Could you check a few things on this model? Use its own coordinates, in mm. Face numbers are marked on the shaded views. A direction names the side the tool comes from. Round coordinates to 2 decimals unless told otherwise and drop trailing zeros. Write each loop counter-clockwise with the first axis right and the second up, starting at its lowest first coordinate (ties: lowest second). Pieces come first, ordered by that corner, then holes. Notation, with made-up numbers: M -18,-2.75 L 10,-2.75 A29 cw 10,18.25 Z; hole C 24.5,-3.75 d10. An arc over 180 degrees is marked long. One line per question, with ' | ' between items. Start each with the question number.
```python
from build123d import *

# Parameters (mm, degrees)
F2_R    = 0.5
F3_R    = 0.9
F4_SIZE = 0.5


with BuildPart() as f1:
    # F0 (on Front) → F1 (revolve)
    with BuildSketch(Plane.XZ):
        with BuildLine():
            ThreePointArc((0, 0.7), (5.511125, 0.524823), (11, 0))
            Line((11, 0), (11, 2))
            Line((11, 2), (5.55, 2))
            Line((5.55, 2), (5.55, 2.45))
            Line((5.55, 2.45), (2.55, 2.45))
            Line((2.55, 2.45), (4.05, 3.95))
            Line((4.05, 3.95), (4.05, 5.75))
            Line((4.05, 5.75), (0, 5.75))
            Line((0, 5.75), (0, 0.7))
        make_face()
    revolve(axis=Axis((0, 0, 3.225), (0, 0, -1)))

    # F2
    f2_edges = [f1.edges().sort_by_distance(p)[0] for p in [
        (-2.55, 0, 2.45),
    ]]
    fillet(f2_edges, radius=F2_R)

    # F3
    f3_edges = [f1.edges().sort_by_distance(p)[0] for p in [
        (-11, 0, 0),
        (-11, 0, 2),
    ]]
    fillet(f3_edges, radius=F3_R)

    # F4
    f4_edges = [f1.edges().sort_by_distance(p)[0] for p in [
        (-4.05, 0, 5.75),
    ]]
    chamfer(f4_edges, length=F4_SIZE)


solid = f1.part
```
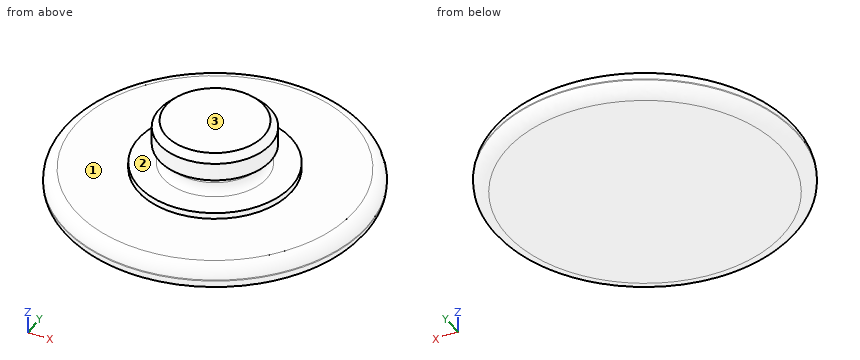
1. I need wall thicknesses on line 1 along Z through (x, y) = (-6.75, 7.5); line 2 along Y through (x, z) = (3.75, 2.2); line 3 along Z through (x, y) = (7.25, -8). Which ranges of each line are inside material? Lowest first, please. Write a range as from..to.
2. Suppose I cut it at B-B (z = 2.8). Write out the boundary of the cut face in (x, y).
3. Which directions (+Z, -Z, +X, -X, +Y, -Y) give clear straight access to the entire face, cutting with the end or side of a thin tool? Please do the marked faces 1, 2 and 3.
4. I'm going to push flat-ended pins straight in: P1, Ø1.5, axis at x = -6.5, y = -8, coming from the +Z side; P2, Ø3, axis at x = 3, y = -4.5, coming from the +Z side. Where does each tip first touch, or does it pass through?
5. Suppose I cut it at A-A (z = 4.6). Write out the boundary of the cut face in (x, y), and give its area (3 significant figures).
Computed:
1) line 1: z = 0.12..2 | line 2: y = -4.09..4.09 | line 3: z = 0.45..1.67
2) outline: C 0,0 d6.56
3) face 1: +Z | face 2: none | face 3: +Z, +X, -X, +Y, -Y
4) P1: stops at z = 2 | P2: stops at z = 5.39
5) outline: C 0,0 d8.1 | area: 51.5 mm²
